Input: part model. Units: mm. Frame: model coordinates. A direction names the side the tool comes from. Coordinates: 2 decimals unless noted, no trailing zeros. Loops run counter-clockwise (first coordinate to the right, second up) from the corner with the lowest first, then second, coordinate; pieces in that order, holes last.
```python
from build123d import *

# Parameters (mm, degrees)
SKETCH1_W           = 100
SKETCH1_H           = 30
SKETCH1_R           = 2.5
SKETCH1_W_2         = 52
SKETCH1_H_2         = 27
BOSS_EXTRUDE1_DEPTH = 4
SKETCH2_W           = 4
SKETCH2_H           = 4
SKETCH2_R           = 1
BOSS_EXTRUDE2_DEPTH = 2.5


with BuildPart() as part:
    # Sketch1 → Boss-Extrude1 (new body)
    with BuildSketch(Plane.XY):
        Rectangle(SKETCH1_W, SKETCH1_H)
        with Locations((-40, 0)):
            Circle(SKETCH1_R, mode=Mode.SUBTRACT)
        with Locations((40, 0)):
            Circle(SKETCH1_R, mode=Mode.SUBTRACT)
        Rectangle(SKETCH1_W_2, SKETCH1_H_2, mode=Mode.SUBTRACT)
    extrude(amount=BOSS_EXTRUDE1_DEPTH)

    # Sketch2 → Boss-Extrude2 (add)
    with BuildSketch(Plane.XY):
        with Locations((24, -11.5)):
            Rectangle(SKETCH2_W, SKETCH2_H)
        with Locations((23.6, -11.1)):
            Circle(SKETCH2_R, mode=Mode.SUBTRACT)
        with Locations((24, 11.5)):
            Rectangle(SKETCH2_W, SKETCH2_H)
        with Locations((23.6, 11.1)):
            Circle(SKETCH2_R, mode=Mode.SUBTRACT)
        with Locations((-24, -11.5)):
            Rectangle(SKETCH2_W, SKETCH2_H)
        with Locations((-23.6, -11.1)):
            Circle(SKETCH2_R, mode=Mode.SUBTRACT)
        with Locations((-24, 11.5)):
            Rectangle(SKETCH2_W, SKETCH2_H)
        with Locations((-23.6, 11.1)):
            Circle(SKETCH2_R, mode=Mode.SUBTRACT)
    extrude(amount=BOSS_EXTRUDE2_DEPTH)


solid = part.part
```
Item 1: Section query C-C (y = 0). Output: boundary loops of the cut face in (x, z), then the cut area to 3 significant figures.
Result:
outline: (-50, 0) - (-42.5, 0) - (-42.5, 4) - (-50, 4) - close; (-37.5, 0) - (-26, 0) - (-26, 4) - (-37.5, 4) - close; (26, 0) - (37.5, 0) - (37.5, 4) - (26, 4) - close; (42.5, 0) - (50, 0) - (50, 4) - (42.5, 4) - close
area: 152 mm2
Item 2: Section query B-B (x = 1). Output: boundary loops of the cut face in (y, z).
Result:
outline: (-15, 0) - (-13.5, 0) - (-13.5, 4) - (-15, 4) - close; (13.5, 0) - (15, 0) - (15, 4) - (13.5, 4) - close
Item 3: Section query D-D (z = 1.6). Output: boundary loops of the cut face in (x, y).
Result:
outline: (-50, -15) - (50, -15) - (50, 15) - (-50, 15) - close; hole circle Ø5 at (-40, 0); hole (-26, -9.5) - (-22, -9.5) - (-22, -13.5) - (22, -13.5) - (22, -9.5) - (26, -9.5) - (26, 9.5) - (22, 9.5) - (22, 13.5) - (-22, 13.5) - (-22, 9.5) - (-26, 9.5) - close; hole circle Ø2 at (-23.6, -11.1); hole circle Ø2 at (-23.6, 11.1); hole circle Ø2 at (23.6, -11.1); hole circle Ø2 at (23.6, 11.1); hole circle Ø5 at (40, 0)
Item 4: Reachability of faces 1 (the face through (-24.5, -11.9, 2.5)), 2 (the face through (-1, 14, 4)), 3 (the face through (24, -9.5, 1)) from +Z, -Z, +X, -X, +Y, -Y: full face, straight path, thin tool, end or side. Return the list, or none.
Result:
face 1: +Z
face 2: +Z, +X, -X, +Y, -Y
face 3: +Z, -Z
Item 5: Mould query, pull axis Y, two halves, no side actions, for faces 4 (the face through (-1, 15, 2)), 5 (the face through (-24.5, 12, 2.5)), 6 (the face through (-1, 14, 0)). Classes: +Y half, -Y half, draft (parallel to the pull), parting line (faces both ways), or undercut.
Result:
face 4: +Y half
face 5: undercut
face 6: draft
Item 6: Contact query for a flat-ended pin moving along its axis: P1, Ø12, axis at x = 34.5, y = 8, coming from the -Z side. Output: stop coordinate, or through.
Result:
P1: stops at z = 0
Item 7: Line query: L1, parallel to X at y = 11, z = 0.7; L2, parallel to Y at x = -23.6, z = 0.8; L3, parallel to Y at x = -6, z = 2. Output: solid intervals per line, ascending.
Result:
L1: x = -50 to -24.59, -22.61 to -22, 22 to 22.61, 24.59 to 50
L2: y = -15 to -12.1, -10.1 to -9.5, 9.5 to 10.1, 12.1 to 15
L3: y = -15 to -13.5, 13.5 to 15
Item 8: Section query A-A (x = 23.6). Output: boundary loops of the cut face in (y, z).
Result:
outline: (-15, 0) - (-12.1, 0) - (-12.1, 2.5) - (-13.5, 2.5) - (-13.5, 4) - (-15, 4) - close; (-10.1, 0) - (-9.5, 0) - (-9.5, 2.5) - (-10.1, 2.5) - close; (9.5, 0) - (10.1, 0) - (10.1, 2.5) - (9.5, 2.5) - close; (12.1, 0) - (15, 0) - (15, 4) - (13.5, 4) - (13.5, 2.5) - (12.1, 2.5) - close
